from build123d import *

# Parameters (mm, degrees)
F0_W     = 500
F0_H     = 700
F0_W_2   = 470
F0_H_2   = 670
F1_DEPTH = 15
F2_W     = 500
F2_H     = 700
F3_DEPTH = 3


with BuildPart() as f1:
    # F0 (on Front) → F1 (new body)
    with BuildSketch(Plane.XZ):
        with Locations((3.746569, 20.465286)):
            Rectangle(F0_W, F0_H)
        with Locations((3.746569, 20.465286)):
            Rectangle(F0_W_2, F0_H_2, mode=Mode.SUBTRACT)
    extrude(amount=F1_DEPTH)

    # F2 (on face) → F3 (join)
    with BuildSketch(Plane.XZ.offset(15)):
        with Locations((3.746569, 20.465286)):
            Rectangle(F2_W, F2_H)
    extrude(amount=F3_DEPTH)


solid = f1.part
Input: part model. Units: mm. Frame: model coordinates. A direction names the side the tool comes from. Give positions to 0.01 mm unless a question says otherwise; leave off trailing zeros. Loops run counter-clockwise (first coordinate to the right, second up) from the corner with the lowest first, then second, coordinate; pieces in that order, holes last. Notation, with made-up numbers: (-1, 51) -> (46, 51) arc R5 ccw to (46, 59) -> close; hole circle Ø4 at (35.5, -34). An arc over 180 degrees is marked (long way). Answer as a JSON object with one key per item and string values. Group by question number.
Item 1: Line query: probe 1 along Z at (x, y) = (-172, -10.5); probe 2 along X at (y, z) = (-8.5, 113); probe 3 along Y at (x, z) = (-132, -285). Output: solid intervals per line, ascending.
Item 2: Cut plane B-B, the plane x = 46.5. Return the cut outline in (y, z), and give its area (3 significant figures).
Item 3: Pull-direction query (X, two-part tool) for faces 1 (the flat face through (0, -18, 25)), 2 (the flat face through (0, -15, 25)), 3 (the flat face through (-246.253, -9, 16)), 4 (the flat face through (253.747, -9, 16)); classes: released by +X, released by -X, zero draft, split by the parting line, or undercut.
Item 4: Reachability of faces 5 (the flat face through (0, -7, 355.465)), 6 (the flat face through (0, -9, 370.465)) from +Z, -Z, +X, -X, +Y, -Y: full face, straight path, thin tool, end or side. Return the list, or none.
Item 5: Cut plane A-A, the plane y = -4. Return the cut outline in (x, z).
Item 6: Cut plane C-C, the plane z = -71. Return the cut outline in (x, y).
Checks:
{
 "1": {"probe 1": "z = -329.53 to -314.53, 355.47 to 370.47", "probe 2": "x = -246.25 to -231.25, 238.75 to 253.75", "probe 3": "y = -18 to -15"},
 "2": {"outline": "(-18, -329.53) -> (0, -329.53) -> (0, -314.53) -> (-15, -314.53) -> (-15, 355.47) -> (0, 355.47) -> (0, 370.47) -> (-18, 370.47) -> close", "area": "2,550 mm²"},
 "3": {"face 1": "zero draft", "face 2": "undercut", "face 3": "released by -X", "face 4": "released by +X"},
 "4": {"face 5": "+Y", "face 6": "+Z, +X, -X, +Y, -Y"},
 "5": {"outline": "(-246.25, -329.53) -> (253.75, -329.53) -> (253.75, 370.47) -> (-246.25, 370.47) -> close; hole (-231.25, -314.53) -> (238.75, -314.53) -> (238.75, 355.47) -> (-231.25, 355.47) -> close"},
 "6": {"outline": "(-246.25, -18) -> (253.75, -18) -> (253.75, 0) -> (238.75, 0) -> (238.75, -15) -> (-231.25, -15) -> (-231.25, 0) -> (-246.25, 0) -> close"}
}
